Read the model definition and answer for the solid it produces. Units are mm, in the model's axes. A direction names the side the tool comes from. Coordinates: 2 decimals unless noted, no trailing zeros. Loops run counter-clockwise (first coordinate to the right, second up) from the corner with the lowest first, then second, coordinate; pieces in that order, holes last. Notation, with made-up numbers: (-38.5, 18.25) -> (1.5, 18.25) arc R37 ccw to (1.5, 54.25) -> close; hole circle Ø7 at (73.25, 87). An arc over 180 degrees is marked (long way). Answer as a JSON object with one key per item and string values. Group by question number.
Q1. The part is cut by section B-B on z = -23.5. Write down the section's boundary in (x, y), and give its area (3 significant figures).
Q2. Each of these flat-tipped pins is pushed along its axis until it touches: P1, Ø1, axis at x = 67, z = 28, coming from the +Y side; P2, Ø5, axis at x = 62, y = 32, coming from the -Z side; P3, Ø1.5, axis at y = -2, z = -16.5, coming from the +X side; P4, Ø10, axis at y = 9.5, z = 47.5, coming from the +X side. Where does it stop, or does it pass through?
Q3. The part is cut by section A-A on y = 65. Write down the section's boundary in (x, z), and give its area (3 significant figures).
Q4. The part is cut by section D-D on z = 0. Write down the section's boundary in (x, y), and give its area (3 significant figures).
Q5. The part is cut by section C-C on x = 73.5. Write down the section's boundary in (y, z), and give its area (3 significant figures).
Q6. Straight lines are drawn through the part: line 1 along Y through (x, z) = (-12, -10); line 2 along Z through (x, y) = (58, 42); line 3 along Z through (x, y) = (52.5, 50.5). For each, find the intervals that lie inside material, in ascending order. Write a range as [from, to].
Q7. For faces 5 (the flat face through (43.57, -1.48, -74.07)), 6 (the flat face through (-42.36, -1.48, -74.77)), 7 (the flat face through (-40, -3, -77)), 8 (the flat face through (-43.57, -1.48, 74.07)), determine the directions among +Z, -Z, +X, -X, +Y, -Y from which every point of the face is accessible in a straight line to the end or side of a thin tool.
Q8. Determine the mould class of faces 1 (the flat face through (-44.83, -4.014, 79.117)), 2 (the cylindrical face through (64.583, 37.045, 2.283)), 3 (the flat face through (1, -5, 1)), 4 (the flat face through (44.83, -4.014, -79.117)) for opening direction X: released by +X, released by -X, zero draft, split by the parting line, or undercut.
Autodesk Inventor part; units mm, degrees
ref_plane "Work Plane1" through (-38.9815, 70, 0) normal (1, 0, 0) x (0, 1, 0)
ref_plane "XZ Plane" through (0, 0, 0) normal (0, 1, 0) x (-1, 0, 0)
sketch "Sketch2" plane through (0, 0, 0) normal (0, 0, 1) x (1, 0, 0)
  line L0 (0, 0) -> (-38.9815, 0)
  line L1 (-46.3001, 0) -> (-38.9815, 0)
  line L2 (-38.9815, 0) -> (-31.6629, 0)
  line L3 (-49.7315, 70) -> (-64.9343, 70)
  line L4 (-64.9343, 70) -> (-64.9343, 0)
  line L5 (-64.9343, 0) -> (-49.7315, 0)
  line L6 (-49.7315, 0) -> (-49.7315, 70)
  line L7 (-38.9815, 70) -> (-38.9815, 0) construction
  line L8 (-57.3329, 70) -> (-57.3329, 0)
  dimension "d1" = 38.9815
  dimension "d53" = 70
sketch "Sketch3" plane through (0, 0, 0) normal (0, 1, 0) x (-1, 0, 0)
  circle A0 centre (0, 0) radius 105
  circle A1 centre (38.9815, 0) radius 7.3186
  line L0 (0, -105) -> (-90.9327, -52.5)
  line L1 (-90.9327, -52.5) -> (-90.9327, 52.5)
  line L2 (-90.9327, 52.5) -> (0, 105)
  line L3 (0, 105) -> (90.9327, 52.5)
  line L4 (90.9327, 52.5) -> (90.9327, -52.5)
  line L5 (90.9327, -52.5) -> (0, -105)
  line L6 (-85.9327, -49.6132) -> (0, -99.2265)
  line L7 (0, -99.2265) -> (85.9327, -49.6132)
  line L8 (85.9327, -49.6132) -> (85.9327, 49.6132)
  line L9 (85.9327, 49.6132) -> (0, 99.2265)
  line L10 (0, 99.2265) -> (-85.9327, 49.6132)
  line L11 (-85.9327, 49.6132) -> (-85.9327, -49.6132)
  dimension "d14" = 210
  dimension "d15" = 5
extrude "Extrusion3" add sketch "Sketch3" against normal blind 5 contours A1 | L11 L10 L9 L8 L7 L6
extrude "Extrusion4" add sketch "Sketch3" along normal blind 2 from surface at -5 contours L4 L5 L0 L1 L2 L3
sketch "Sketch7" plane through (0, 0, 0) normal (0, 1, 0) x (-1, 0, 0)
  circle A0 centre (57.3329, 0) radius 7.6014
  line L0 (64.9343, 0) -> (49.7315, 0)
  point P0 (0, 0)
  point P1 (64.9343, 0)
  point P2 (64.9343, 0)
  point P3 (49.7315, 0)
sweep "Sweep1" add profiles "Sketch7" path "Sketch2" path curves L8
ref_plane "Work Plane1" through (-38.9815, 70, 0) normal (1, 0, 0) x (0, 1, 0)
sketch "Sketch8" plane through (-38.9815, 70, 0) normal (1, 0, 0) x (0, 1, 0)
  point P0 (-70, 0)
sketch "Sketch10" plane through (-38.9815, 70, 0) normal (1, 0, 0) x (0, 1, 0)
  line L0 (0, 0) -> (-25, 0) construction
  circle A0 centre (-25, 0) radius 5.5
  circle A1 centre (-25, 0) radius 9.5
  circle A2 centre (0, 0) radius 25 construction
  circle A3 centre (-19.2628, 15.9356) radius 9.5
  circle A4 centre (-19.2628, 15.9356) radius 5.5
  circle A5 centre (-4.6845, 24.5572) radius 9.5
  circle A6 centre (-4.6845, 24.5572) radius 5.5
  circle A7 centre (12.0438, 21.9077) radius 9.5
  circle A8 centre (12.0438, 21.9077) radius 5.5
  circle A9 centre (23.2444, 9.2031) radius 9.5
  circle A10 centre (23.2444, 9.2031) radius 5.5
  circle A11 centre (23.7764, -7.7254) radius 9.5
  circle A12 centre (23.7764, -7.7254) radius 5.5
  point P0 (-70, 0)
  dimension "d38" = 11
  dimension "d39" = 4
  dimension "d42" = 198
  dimension "d49" = 25
extrude "Extrusion9" [suppressed]
fillet "Fillet5" radius 5 1 edges at (-64.9343, 0, 0)
mirror "Mirror4" about plane through (0, 0, 0) normal (1, 0, 0) of "Sweep1", "Fillet5"
equation "\"d1\" = 0.5 * ballDist"
equation "\"ballDist\" = 77.963"
equation "\"ballDiam\" = 12.7"
equation "\"clearance\" = 0.4"
properties part number "mounter"
Final values:
{
 "1": {"outline": "(-90.93, -5) -> (90.93, -5) -> (90.93, -3) -> (85.93, -3) -> (85.93, 0) -> (-85.93, 0) -> (-85.93, -3) -> (-90.93, -3) -> close", "area": "879 mm2"},
 "2": {"P1": "stops at y = 0", "P2": "stops at z = -7.29", "P3": "stops at x = 85.93", "P4": "passes through"},
 "3": {"outline": "circle Ø15.2 at (-57.33, 0); circle Ø15.2 at (57.33, 0)", "area": "363 mm2"},
 "4": {"outline": "(-90.93, -5) -> (90.93, -5) -> (90.93, -3) -> (85.93, -3) -> (85.93, 0) -> (69.93, 0) arc R5 cw to (64.93, 5) -> (64.93, 70) -> (49.73, 70) -> (49.73, 5) arc R5 cw to (44.73, 0) -> (-44.73, 0) arc R5 cw to (-49.73, 5) -> (-49.73, 70) -> (-64.93, 70) -> (-64.93, 5) arc R5 cw to (-69.93, 0) -> (-85.93, 0) -> (-85.93, -3) -> (-90.93, -3) -> close", "area": "3,030 mm2"},
 "5": {"outline": "(-5, -62.56) -> (-3, -62.56) -> (-3, -56.79) -> (0, -56.79) -> (0, 56.79) -> (-3, 56.79) -> (-3, 62.56) -> (-5, 62.56) -> close", "area": "591 mm2"},
 "6": {"line 1": "y = [-5, 0]", "line 2": "z = [-7.57, 7.57]", "line 3": "z = [-5.87, 5.87]"},
 "7": {"face 5": "-Z, +X, +Y", "face 6": "-Z, -X, +Y", "face 7": "+Y", "face 8": "+Z, -X, +Y"},
 "8": {"face 1": "released by -X", "face 2": "undercut", "face 3": "zero draft", "face 4": "released by +X"}
}
